Autodesk Inventor part; units mm, degrees
ref_plane "Work Plane1" through (-15, 15, 7) normal (0, 0, 1) x (1, 0, 0)
ref_plane "Work Plane2" through (-15, 15, -5.5) normal (0, 0, 1) x (1, 0, 0)
ref_plane "YZ Plane" through (0, 0, 0) normal (1, 0, 0) x (0, 1, 0)
sketch "Sketch1" plane through (0, 0, 0) normal (0, 0, 1) x (1, 0, 0)
  line L0 (0, 0) -> (-75, 0)
  line L1 (0, 0) -> (0, 50)
  line L2 (0, 50) -> (-38, 50)
  line L3 (-75, 0) -> (-75, 5)
  spline S0 degree 3 poles (-38, 50) (-46.7224, 6.6996) (-125.1064, 18.5226) (-28.5296, -55.0422) knots 0 0 0 0 1 1 1 1
  point P0 (-58.1914, 22.009)
  dimension "d0" = 75
  dimension "d1" = 50
  dimension "d2" = 38
  dimension "d3" = 5
revolve "Revolution1" add sketch "Sketch1" angle 360 about axis through (0, 0, 0) along (0, 1, 0)
sketch "Sketch2" plane through (0, 50, 0) normal (0, 1, 0) x (1, 0, 0)
  line L0 (-15, 24) -> (15, 24)
  line L1 (15, 24) -> (15, -24)
  line L2 (15, -24) -> (-15, -24)
  line L3 (-15, -24) -> (-15, 24)
  point P0 (0, 0)
  dimension "d5" = 30
  dimension "d6" = 48
  dimension "d7" = 24
  dimension "d8" = 15
extrude "Extrusion1" cut sketch "Sketch2" against normal blind 35
sketch "Sketch3" plane through (0, 15, 0) normal (0, 1, 0) x (1, 0, 0)
  line L0 (15, -24) -> (-15, -24)
  line L1 (-15, -24) -> (-15, 24)
  line L2 (15, -24) -> (-15, -24)
  line L3 (-15, -24) -> (-15, -7)
  line L4 (-15, -7) -> (15, -7)
  line L5 (15, -7) -> (15, -24)
  point P0 (0, 0)
  dimension "d11" = 17
extrude "Extrusion2" cut sketch "Sketch3" against normal blind 8
sketch "Sketch4" plane through (0, 0, 0) normal (0, 0, 1) x (1, 0, 0)
  circle A0 centre (-26, 38) radius 2.6
  circle A1 centre (-53, 12) radius 2.6
  line L0 (75, 0) -> (-75, 0)
  line L1 (38, 50) -> (-38, 50)
  line L2 (-75, 0) -> (-75, 5)
  line L3 (15, 50) -> (-15, 50) construction
  line L4 (0, 50) -> (0, 20.8019) construction
  circle A2 centre (26, 38) radius 2.6
  circle A3 centre (53, 12) radius 2.6
  point P0 (0, 0)
  dimension "d14" = 5.2
  dimension "d15" = 5.2
  dimension "d16" = 12
  dimension "d17" = 12
  dimension "d18" = 22
  dimension "d19" = 12
extrude "Extrusion3" cut sketch "Sketch4" along normal blind 52 and the other way blind 52
ref_plane "Work Plane1" through (-15, 15, 7) normal (0, 0, 1) x (1, 0, 0)
split "Split1" plane through (-15, 15, 7) removes the side toward (0, 0, 1)
sketch "Sketch6" plane through (0, 0, 0) normal (0, -1, 0) x (1, 0, 0)
  circle A0 centre (0, 0) radius 10.5
  dimension "d25" = 21
extrude "Extrusion4" cut sketch "Sketch6" against normal blind 2.5
ref_plane "Work Plane2" through (-15, 15, -5.5) normal (0, 0, 1) x (1, 0, 0)
sketch "Sketch7" plane through (-15, 15, -5.5) normal (0, 0, 1) x (1, 0, 0)
  circle A0 centre (41, 23) radius 2.6
  line L0 (38.6906, 27) -> (43.3094, 27)
  line L1 (43.3094, 27) -> (45.6188, 23)
  line L2 (45.6188, 23) -> (43.3094, 19)
  line L3 (43.3094, 19) -> (38.6906, 19)
  line L4 (38.6906, 19) -> (36.3812, 23)
  line L5 (36.3812, 23) -> (38.6906, 27)
  circle A1 centre (-11, 23) radius 2.6
  line L6 (-13.3094, 27) -> (-8.6906, 27)
  line L7 (-8.6906, 27) -> (-6.3812, 23)
  line L8 (-6.3812, 23) -> (-8.6906, 19)
  line L9 (-8.6906, 19) -> (-13.3094, 19)
  line L10 (-13.3094, 19) -> (-15.6188, 23)
  line L11 (-15.6188, 23) -> (-13.3094, 27)
  circle A2 centre (-38, -3) radius 2.6
  line L12 (-35.6906, 1) -> (-33.3812, -3)
  line L13 (-33.3812, -3) -> (-35.6906, -7)
  line L14 (-35.6906, -7) -> (-40.3094, -7)
  line L15 (-40.3094, -7) -> (-42.6188, -3)
  line L16 (-42.6188, -3) -> (-40.3094, 1)
  line L17 (-40.3094, 1) -> (-35.6906, 1)
  circle A3 centre (68, -3) radius 2.6
  line L18 (65.6906, 1) -> (70.3094, 1)
  line L19 (70.3094, 1) -> (72.6188, -3)
  line L20 (72.6188, -3) -> (70.3094, -7)
  line L21 (70.3094, -7) -> (65.6906, -7)
  line L22 (65.6906, -7) -> (63.3812, -3)
  line L23 (63.3812, -3) -> (65.6906, 1)
  line L24 (30, 35) -> (52.3497, 35)
  line L25 (-22.3497, 35) -> (0, 35)
  point P0 (15, -15)
  dimension "d29" = 8
  dimension "d30" = 8
  dimension "d31" = 8
  dimension "d32" = 8
extrude "Extrusion5" cut sketch "Sketch7" against normal blind 50 contours A0 | L0 L1 L2 L3 L4 L5 | A1 | L6 L7 L8 L9 L10 L11 | A2 | L12 L13 L14 L15 L16 L17 | A3 | L18 L19 L20 L21 L22 L23
sketch "Sketch8" plane through (-15, 15, 7) normal (0, 0, 1) x (1, 0, 0)
  point P0 (15, -15)
sketch "Sketch9" plane through (-15, 15, 7) normal (0, 0, 1) x (1, 0, 0)
  arc A0 (8.3697, -6.5166) -> (4.6303, -6.5166) centre (6.5, -4.5) ccw
  arc A1 (25.3697, -6.5166) -> (22.2084, -6.9278) centre (23.5, -4.5) ccw
  circle A2 centre (6.5, -4.5) radius 4.25
  circle A3 centre (23.5, -4.5) radius 4.25
  line L0 (7.1738, -15) -> (-59.6726, -15)
  spline S0 degree 3 poles (-59.6726, -10) (-58.7689, -7.9323) (-57.4468, -6.0708) (-54.3242, -2.5217) (-52.3894, -0.7667) (-46.4805, 4.2144) (-41.726, 7.6418) (-33.4997, 14.92) (-30.0416, 18.5511) (-24.9099, 26.5974) (-23.2478, 30.6178) (-22.3497, 35) knots -6.163162 -6.163162 -6.163162 -6.163162 -5.426539 -5.426539 -4.614235 -4.614235 -2.856788 -2.856788 -1.341997 -1.341997 0 0 0 0
  line L1 (-59.6726, -15) -> (-59.6726, -10)
  line L2 (-22.3497, 35) -> (0, 35)
  spline S1 degree 3 poles (52.3497, 35) (53.0647, 31.5111) (54.27, 28.2261) (57.5622, 22.1809) (59.5109, 19.5298) (66.0487, 12.2093) (71.1762, 8.2595) (79.7672, 1.4925) (83.3346, -1.3766) (87.4881, -6.1291) (88.7829, -7.9645) (89.6726, -10) knots -5.079654 -5.079654 -5.079654 -5.079654 -4.231884 -4.231884 -3.44283 -3.44283 -1.900227 -1.900227 -0.666449 -0.666449 0 0 0 0
  line L3 (30, 35) -> (52.3497, 35)
  line L4 (89.6726, -10) -> (89.6726, -15)
  line L5 (89.6726, -15) -> (22.8262, -15)
  point P0 (15, -15)
  dimension "d35" = 8.5
  dimension "d36" = 8.5
extrude "Extrusion6" cut sketch "Sketch9" against normal blind 1
sketch "Sketch10" plane through (-8.5, 10.5, 6) normal (0, 0, 1) x (1, 0, 0)
  circle A0 centre (0, 0) radius 0.75
  circle A1 centre (17, 0) radius 4.25
  circle A2 centre (17, 0) radius 0.75
  point P0 (8.5, -10.5)
  dimension "d39" = 1.5
  dimension "d40" = 1.5
extrude "Extrusion7" cut sketch "Sketch10" against normal blind 10 contours A0 | A2
properties part number "Podstawa 01-2"
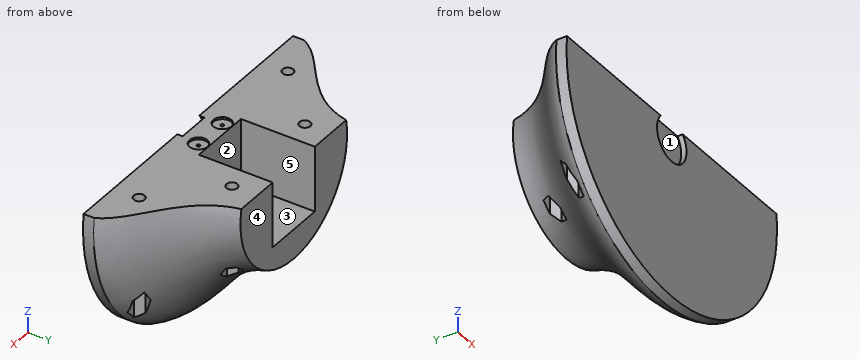
The model under review builds one solid part; all positions refer to its coordinate system, in mm. Face numbers are marked on the shaded views. A direction names the side the tool comes from. Round coordinates to 2 decimals unless told otherwise and drop trailing zeros. Write item = value, one per line. Start each with the question number.
Item 1: Insertion check: pin 1 (1.4 mm diameter, centred on x = -52.5, z = -30.5, fed in from +Y); pin 2 (1.6 mm diameter, centred on x = -8.5, y = 10.5, fed in from +Z); pin 3 (4 mm diameter, centred on x = -52.5, y = 13.5, fed in from -Z). Each pin has a flat end and moves straight along its axis. Give the tip position at first contact, or say it passes through.
Item 2: For the marked faces 4 and 5, list the 3-axis set-ups (+Z, -Z, +X, -X, +Y, -Y) from which the entire face can be reached by the end or side of a thin tool; tool diameter is ignored.
Item 3: Take a section at A-A on z = 0. Count the separate pieces of the cut face and the enclosed holes in it, plus the area to 3 significant figures.
Item 4: To check wall thickness, follow L1, parallel to X at y = 14, z = -33; L2, parallel to Y at x = 8.5, z = 2.25; L3, parallel to X at y = 11, z = -5. State the ranges of each line that lie inside material, in increasing order.
Item 5: Mouldability with a two-part tool opening along Z and no side actions: class the marked faces 1, 2 and 3 as released by +Z, released by -Z, zero draft, split by the parting line, or undercut.
Result:
q1.pin_1 = 20.56
q1.pin_2 = 6
q1.pin_3 = -5.5
q2.face_4 = +Z, -Z, +X, -X, +Y
q2.face_5 = +Z, +Y
q3.separate_pieces = 1
q3.enclosed_holes = 6
q3.area = 4,410 mm²
q4.L1 = -59.4 to -56.46, -49.54 to 49.54, 56.46 to 59.4
q4.L2 = 2.5 to 9.75, 11.25 to 15
q4.L3 = -70.79 to -55.4, -50.6 to 50.6, 55.4 to 70.79
q5.face_1 = undercut
q5.face_2 = zero draft
q5.face_3 = released by +Z
